```python
from build123d import *

# Parameters (mm, degrees)
F1_DEPTH = 63.5
F0_W     = 25.4
F0_H     = 18.905382
F2_DEPTH = 25.4
F3_DEPTH = 7.9375
F5_R     = 6.35


with BuildPart() as f1:
    # F0 (on Front) → F1 (new body, symmetric)
    with BuildSketch(Plane.XZ):
        Polygon((-41.275, -9.525), (41.275, -9.525), (41.275, 9.525), (22.225, 9.525), (-41.275, 9.525), align=None)
    extrude(amount=F1_DEPTH, both=True)

    # F0 (on Front) → F2 (join, symmetric)
    with BuildSketch(Plane.XZ):
        with BuildLine():
            Line((22.225, 9.525), (41.275, 9.525))
            Line((41.275, 9.525), (41.275, 27.0002))
            ThreePointArc((41.275, 27.0002), (45.92468, 38.22552), (57.15, 42.8752))
            Line((57.15, 42.8752), (60.325, 42.8752))
            Line((60.325, 42.8752), (60.325, 61.780582))
            add(Edge.make_bspline(
                [(54.418618, 61.818229), (56.398661, 61.826097), (58.368865, 61.812328), (60.325, 61.780582)],
                knots=[108.678024, 108.678024, 108.678024, 108.678024, 114.250628, 114.250628, 114.250628, 114.250628], degree=3))
            ThreePointArc((54.418618, 61.818229), (31.506783, 50.710557), (22.225, 27.0002))
            Line((22.225, 27.0002), (22.225, 9.525))
        make_face()
        with Locations((73.025, 52.327891)):
            Rectangle(F0_W, F0_H)
    extrude(amount=F2_DEPTH, both=True)

    # F0 (on Front) → F3 (join, symmetric)
    with BuildSketch(Plane.XZ):
        with BuildLine():
            add(Edge.make_bspline(
                [(-41.275, 9.525), (-26.553893, 53.282353), (15.803419, 61.664801), (54.418618, 61.818229)],
                knots=[0, 0, 0, 0, 108.678024, 108.678024, 108.678024, 108.678024], degree=3))
            Line((-41.275, 9.525), (22.225, 9.525))
            Line((22.225, 9.525), (22.225, 27.0002))
            ThreePointArc((22.225, 27.0002), (31.506783, 50.710557), (54.418618, 61.818229))
        make_face()
    extrude(amount=F3_DEPTH, both=True)

    # F0 (on Front) → F4 (revolve)
    with BuildSketch(Plane.XZ):
        Polygon((85.725, 66.675), (85.725, 61.780582), (85.725, 42.8752), (85.725, 38.1), (111.125, 38.1), (111.125, 66.675), align=None)
    revolve(axis=Axis((85.725, 0, 52.3875), (0, 0, 1)))

    # F5
    f5_edges = [f1.edges().sort_by_distance(p)[0] for p in [
        (41.275, -63.5, 0),
        (-41.275, -63.5, 0),
        (-41.275, 63.5, 0),
        (41.275, 63.5, 0),
    ]]
    fillet(f5_edges, radius=F5_R)


solid = f1.part
```
Geometry check sheet. Reference: the model listing, model coordinates, mm. A direction names the side the tool comes from. Coordinates: 2 decimals unless noted, no trailing zeros. Order: outer loops, then holes, each group sorted by start corner. A loop starts at its lowest first (then second) coordinate and runs counter-clockwise, first axis right, second up. Notation, with made-up numbers: (65.25, -36) - (105.25, -36) arc R24 cw to (105.25, -3) - close; hole circle Ø3 at (76, -17.5). An arc over 180 degrees is marked (long way). Use one line per item in the form item = value.
1. Scan lines: line 1 (Y direction, x = 21, z = 24.5); line 2 (X direction, y = -47, z = -4.5) (3 decimals); line 3 (Z direction, x = 64, y = 8.5) (3 decimals). Record each from-to range of solid material in increasing order.
Here are the results:
line_1 = -7.94 to 7.94
line_2 = -41.275 to 41.275
line_3 = 38.1 to 66.675
2. Gauge pin test, flat ends, axial feed: pin 1 (1 mm diameter, centred on x = 25, z = 22.5, fed in from +Y); pin 2 (23 mm diameter, centred on x = 77, y = 10, fed in from -Z); pin 3 (6 mm diameter, centred on x = 2, z = 49, fed in from +Y); pin 4 (5 mm diameter, centred on x = 55, y = -29.5, fed in from +Z). Record the tip position at first contact, or that the pin passes through.
Here are the results:
pin_1 = 25.4
pin_2 = 38.1
pin_3 = 7.94
pin_4 = through
3. Section check D-D (x = 89.5). Record the boundary of the cut face in (y, z) (3 decimals).
Here are the results:
outline = (-25.118, 38.1) - (25.118, 38.1) - (25.118, 66.675) - (-25.118, 66.675) - close
4. Section check C-C (y = -43). Record the boundary of the cut face in (x, z) (3 decimals), then the cut area to 3 significant figures.
Here are the results:
outline = (-41.275, -9.525) - (41.275, -9.525) - (41.275, 9.525) - (-41.275, 9.525) - close
area = 1,570 mm²
5. Section check A-A (z = -2). Record the boundary of the cut face in (x, y) (3 decimals).
Here are the results:
outline = (-41.275, -57.15) arc R6.35 ccw to (-34.925, -63.5) - (34.925, -63.5) arc R6.35 ccw to (41.275, -57.15) - (41.275, 57.15) arc R6.35 ccw to (34.925, 63.5) - (-34.925, 63.5) arc R6.35 ccw to (-41.275, 57.15) - close
6. Access from +Z, -Z, +X, -X, +Y, -Y to the whole of each face (thin tool, end or side, straight path). Record for faces 1 (the face through (22.225, 17, 18)), 2 (the face through (85, 0, 66.675)), 3 (the face through (86, 0, 38.1)), 4 (the face through (-3, -7.938, 30)).
Here are the results:
face_1 = +Z, -X, +Y
face_2 = +Z, +X, -X, +Y, -Y
face_3 = -Z, +X, +Y, -Y
face_4 = +Z, -X, -Y
7. Section check B-B (x = 70). Record the boundary of the cut face in (y, z) (3 decimals).
Here are the results:
outline = (-25.4, 42.875) - (-19.947, 42.875) - (-19.947, 38.1) - (19.947, 38.1) - (19.947, 42.875) - (25.4, 42.875) - (25.4, 61.781) - (19.947, 61.781) - (19.947, 66.675) - (-19.947, 66.675) - (-19.947, 61.781) - (-25.4, 61.781) - close
8. Draft check along X on faces 5 (the face through (60, 2, 42.875)), 6 (the face through (31.76, 16.55, 50.98)), 7 (the face through (0, 63.5, 0)). Enter one of: pulls with the +X half, pulls with the -X half, needs draft (parallel to the pull), parting line crosses it, or undercut.
Here are the results:
face_5 = undercut
face_6 = pulls with the -X half
face_7 = needs draft
